```python
from build123d import *

# Parameters (mm, degrees)
SKETCH1_W           = 355.6
SKETCH1_H           = 58.42
BOSS_EXTRUDE1_DEPTH = 4.7625
SKETCH2_W           = 6.858
SKETCH2_H           = 21.806929344
SKETCH2_W_2         = 6.35
SKETCH2_H_2         = 21.298929344
CUT_EXTRUDE1_DEPTH  = 181.246346721
SKETCH3_W           = 1.5875
SKETCH3_H           = 17.817070656
SKETCH3_H_2         = 18.796
CUT_EXTRUDE2_DEPTH  = 181.246346721
SKETCH4_W           = 0.3175
SKETCH4_H           = 21.806929344
BOSS_EXTRUDE2_DEPTH = 4.7625
SKETCH5_W           = 0.3175
SKETCH5_H           = 21.806929344
CUT_EXTRUDE3_DEPTH  = 179.68058278
SKETCH6_R           = 3.429
CUT_EXTRUDE4_DEPTH  = 179.68058278


with BuildPart() as part:
    # Sketch1 → Boss-Extrude1 (new body)
    with BuildSketch(Plane(origin=(0, 0, 0), x_dir=(1, 0, 0), z_dir=(0, 1, 0))):
        Rectangle(SKETCH1_W, SKETCH1_H)
    extrude(amount=BOSS_EXTRUDE1_DEPTH)

    # Sketch2 → Cut-Extrude1 (cut, through all)
    with BuildSketch(Plane(origin=(0, 0, 0), x_dir=(-1, 0, 0), z_dir=(0, -1, 0))):
        with Locations((174.625, 0.489464672)):
            Rectangle(SKETCH2_W, SKETCH2_H)
        with Locations((174.625, 0.489464672)):
            Rectangle(SKETCH2_W_2, SKETCH2_H_2, mode=Mode.SUBTRACT)
        with Locations((79.375, 0.489464672)):
            Rectangle(SKETCH2_W, SKETCH2_H)
        with Locations((79.375, 0.489464672)):
            Rectangle(SKETCH2_W_2, SKETCH2_H_2, mode=Mode.SUBTRACT)
        with Locations((-79.375, 0.489464672)):
            Rectangle(SKETCH2_W, SKETCH2_H)
        with Locations((-79.375, 0.489464672)):
            Rectangle(SKETCH2_W_2, SKETCH2_H_2, mode=Mode.SUBTRACT)
        with Locations((-174.625, 0.489464672)):
            Rectangle(SKETCH2_W, SKETCH2_H)
        with Locations((-174.625, 0.489464672)):
            Rectangle(SKETCH2_W_2, SKETCH2_H_2, mode=Mode.SUBTRACT)
    extrude(amount=-CUT_EXTRUDE1_DEPTH, mode=Mode.SUBTRACT)


with BuildPart() as cut_extrude1_kept_piece:
    # of the separate pieces the step leaves, the one the design keeps (cut_extrude1_pieces_kept)
    add(part.part.solids().sort_by_distance((-177.8, 0, -29.21))[0])

    # Sketch3 → Cut-Extrude2 (cut, through all)
    with BuildSketch(Plane.XZ):
        with Locations((177.00625, -20.301464672)):
            Rectangle(SKETCH3_W, SKETCH3_H)
        with Locations((177.00625, 19.812)):
            Rectangle(SKETCH3_W, SKETCH3_H_2)
        with Locations((-177.00625, -20.301464672)):
            Rectangle(SKETCH3_W, SKETCH3_H)
        with Locations((-177.00625, 19.812)):
            Rectangle(SKETCH3_W, SKETCH3_H_2)
    extrude(amount=-CUT_EXTRUDE2_DEPTH, mode=Mode.SUBTRACT)

    # Sketch4 → Boss-Extrude2 (add)
    with BuildSketch(Plane.XZ):
        with Locations((76.10475, -0.489464672)):
            Rectangle(SKETCH4_W, SKETCH4_H)
        with Locations((-76.10475, -0.489464672)):
            Rectangle(SKETCH4_W, SKETCH4_H)
    extrude(amount=-BOSS_EXTRUDE2_DEPTH)

    # Sketch5 → Cut-Extrude3 (cut, through all)
    with BuildSketch(Plane.XZ):
        with Locations((-82.96275, -0.489464672)):
            Rectangle(SKETCH5_W, SKETCH5_H)
        with Locations((82.96275, -0.489464672)):
            Rectangle(SKETCH5_W, SKETCH5_H)
    extrude(amount=-CUT_EXTRUDE3_DEPTH, mode=Mode.SUBTRACT)

    # Sketch6 → Cut-Extrude4 (cut, through all)
    with BuildSketch(Plane.XZ):
        with Locations(Location((0, 0, 0), (0, 0, 270))):
            Circle(SKETCH6_R)
    extrude(amount=-CUT_EXTRUDE4_DEPTH, mode=Mode.SUBTRACT)


solid = cut_extrude1_kept_piece.part
```
For this review, take the finished solid that the model builds, in its own axes (mm). Coordinates: 2 decimals unless noted, no trailing zeros. Loops run counter-clockwise (first coordinate to the right, second up) from the corner with the lowest first, then second, coordinate; pieces in that order, holes last.
1. Add section B-B, the plane y = 2.7. Give the boundary of the cut face in (x, z).
2. Add section A-A, the plane z = 0. Give the boundary of the cut face in (x, y).
3. For line 1 (X direction, y = 2.3, z = 0); line 2 (X direction, y = 0.5, z = -3); line 3 (Z direction, x = -1, y = 1.4), list the stretches that pass through material, from the lowest coordinate up.
4. Insertion check: P1, Ø1.4, axis at y = 2, z = -0.5, coming from the +X side; P2, Ø2.5, axis at y = 3.5, z = -1.5, coming from the -X side. Each pin has a flat end and moves straight along its axis. Give the tip position at first contact, or say it passes through.
5. Mouldability with a two-part tool opening along Z and no side actions: class faces 1 (the cylindrical face through (-3.35, 2.35, 0.74)), 2 (the flat face through (-2, 0, -6)) as +Z half, -Z half, draft (parallel to the pull), parting line (faces both ways), or undercut.
Result:
1. outline: (-176.21, -29.21) - (176.21, -29.21) - (176.21, -11.39) - (171.2, -11.39) - (171.2, 10.41) - (176.21, 10.41) - (176.21, 29.21) - (-176.21, 29.21) - (-176.21, 10.41) - (-171.2, 10.41) - (-171.2, -11.39) - (-176.21, -11.39) - close; hole (-83.12, -11.39) - (-76.26, -11.39) - (-76.26, 10.41) - (-83.12, 10.41) - close; hole circle Ø6.86 at (0, 0); hole (76.26, -11.39) - (83.12, -11.39) - (83.12, 10.41) - (76.26, 10.41) - close
2. outline: (-171.2, 0) - (-83.12, 0) - (-83.12, 4.76) - (-171.2, 4.76) - close; (-76.26, 0) - (-3.43, 0) - (-3.43, 4.76) - (-76.26, 4.76) - close; (3.43, 0) - (76.26, 0) - (76.26, 4.76) - (3.43, 4.76) - close; (83.12, 0) - (171.2, 0) - (171.2, 4.76) - (83.12, 4.76) - close
3. line 1: x = -171.2 to -83.12, -76.26 to -3.43, 3.43 to 76.26, 83.12 to 171.2
3. line 2: x = -171.2 to -83.12, -76.26 to -1.66, 1.66 to 76.26, 83.12 to 171.2
3. line 3: z = -29.21 to -3.28, 3.28 to 29.21
4. P1: stops at x = 171.2
4. P2: stops at x = -171.2
5. face 1: undercut
5. face 2: draft
